Part model, mm, in its own coordinate system. Give positions to 0.01 mm unless a question says otherwise; leave off trailing zeros. Order: outer loops, then holes, each group sorted by start corner. A loop starts at its lowest first (then second) coordinate and runs counter-clockwise, first axis right, second up. Notation, with made-up numbers: (74.25, 85) - (85.25, 85) arc R18 ccw to (85.25, 97) - close; hole circle Ø4 at (-9, 10). An arc over 180 degrees is marked (long way). Use a Markdown table: item, result. Add a question column.
from build123d import *

# Parameters (mm, degrees)
F1_R     = 24.9577735622
F2_DEPTH = 203.2
F3_D     = 38.1
F3_DEPTH = 127
F3_TIP   = 11.4463947925
F5_D     = 6.35


with BuildPart() as f2:
    # F1 (on Top) → F2 (new body)
    with BuildSketch(Plane.XY):
        Circle(F1_R)
    extrude(amount=F2_DEPTH)

    # F3
    with Locations(Plane(origin=(0, 0, 0), x_dir=(1, 0, 0), z_dir=(0, 0, -1))):
        with Locations((0, 0)):
            Hole(F3_D / 2, depth=F3_DEPTH)
            with Locations((0, 0, -(F3_DEPTH + F3_TIP / 2))):  # 118° drill point
                Cone(0, F3_D / 2, F3_TIP, mode=Mode.SUBTRACT)

    # F5 (through all)
    with Locations(Plane(origin=(0, 0, 0), x_dir=(1, 0, 0), z_dir=(0, 0, -1))):
        with Locations((0, 0)):
            Hole(F5_D / 2)


solid = f2.part
1. Cut at D-D (z = 147). Write the cut outline in (x, y) (3 decimals).
2. Cut at C-C (z = 50). Write the cut outline in (x, y).
3. Drill centre lines: probe 1 along Y at (x, z) = (0, 59); probe 2 along Y at (x, z) = (0, 162) (3 decimals); probe 3 along X at (y, z) = (-7, 95.5). Where is each one in solid material? Low to high. Write a range as [from, to].
4. Cut at A-A (y = 0). Write the cut outline in (x, z) (3 decimals), plus the area to 3 significant figures.
5. Mould opens along Y. For faces 1 (the face through (15.12, 11.59, 64.39)), 2 (the face through (-5.41, -24.364, 100.178)), 3 (the face through (-3.07, -2.82, 135.94)), 4 (the face through (5, 0, 203.2)) say: released by +Y, released by -Y, zero draft, split by the parting line, or undercut.
6. Pin check, flat tips, straight feed: P1, Ø4, axis at y = -1.5, z = 157.5, coming from the +X side; P2, Ø4, axis at x = 18.5, z = 156.5, coming from the -Y side; P3, Ø2, axis at x = -11, y = 9.5, coming from the -Z side; P4, Ø6, axis at x = -13, z = 152, coming from the -Y side. Stop position of each tip, or through.
Responses:
| question | item | result |
|---|---|---|
| 1 | outline | circle Ø49.916 at (0, 0); hole circle Ø6.35 at (0, 0) |
| 2 | outline | circle Ø49.92 at (0, 0); hole circle Ø38.1 at (0, 0) |
| 3 | probe 1 | y = [-24.96, -19.05], [19.05, 24.96] |
| 3 | probe 2 | y = [-24.958, -3.175], [3.175, 24.958] |
| 3 | probe 3 | x = [-23.96, -17.72], [17.72, 23.96] |
| 4 | outline | (-24.958, 0) - (-19.05, 0) - (-19.05, 127) - (-3.175, 136.539) - (-3.175, 203.2) - (-24.958, 203.2) - close; (3.175, 136.539) - (19.05, 127) - (19.05, 0) - (24.958, 0) - (24.958, 203.2) - (3.175, 203.2) - close |
| 4 | area | 4,670 mm² |
| 5 | face 1 | undercut |
| 5 | face 2 | split by the parting line |
| 5 | face 3 | undercut |
| 5 | face 4 | zero draft |
| 6 | P1 | stops at x = 24.96 |
| 6 | P2 | stops at y = -18.73 |
| 6 | P3 | stops at z = 129.11 |
| 6 | P4 | stops at y = -22.87 |
